The figure shows three views and two pictorial views of one solid part (mm, origin at its lowest corner). Answer the questions. A direction names the side the tool comes from. Give positions to 0.01 mm unless a question says otherwise; leave off trailing zeros. Loops run counter-clockwise (first coordinate to the right, second up) from the corner with the lowest first, then second, coordinate; pieces in that order, holes last. Notation, with made-up numbers: (35, 31.5) - (50, 31.5) arc R13 ccw to (50, 41.5) - close; hole circle Ø7 at (-28, -17). An arc over 180 degrees is marked (long way). Use a Markdown table: item, result. Add a question column.
Item 1: Which of the six approach directions +Z, -Z, +X, -X, +Y, -Y give full straight-line access (tool end or side, diameter ignored) to the marked faces 1, 2, 3, 4 and 5?
Item 2: Each of these flat-tipped pins is pushed along its axis until it touches: P1, Ø7.5, axis at x = 29, y = 15.5, coming from the +Z side; P2, Ø3, axis at y = 23, z = 4.5, coming from the +X side; P3, Ø8, axis at y = 25.5, z = 8, coming from the -X side (1 decimal); P4, Ø6.5, axis at x = 42.04, z = 10.16, coming from the -Y side. Where does it stop, or does it pass through?
Item 3: Consider probe 1 along X at (y, z) = (3.5, 10.16); probe 2 along X at (y, z) = (14.75, 16.75) (1 decimal); probe 3 along Y at (x, z) = (39, 16.5). Determine where each line is inside the solid, lowest interval first. Write a range as [from, to].
Item 4: A cutting plane is placed at B-B (x = 44.5). Determine the outline of the cut face in (y, z) (1 decimal), plus the area to 3 significant figures.
Item 5: For a pull along X with two mould halves and no side action, classify the marked faces 6, 7 and 8 as +X half, -X half, draft (parallel to the pull), parting line (faces both ways), or undercut.
Item 6: A cutting plane is placed at C-C (y = 14.25). Determine the outline of the cut face in (x, z) (1 decimal).
Item 7: A cutting plane is placed at D-D (z = 17). Determine the outline of the cut face in (x, y) (1 decimal).
Item 8: A cutting plane is placed at A-A (z = 9). Determine the outline of the cut face in (x, y) (1 decimal).
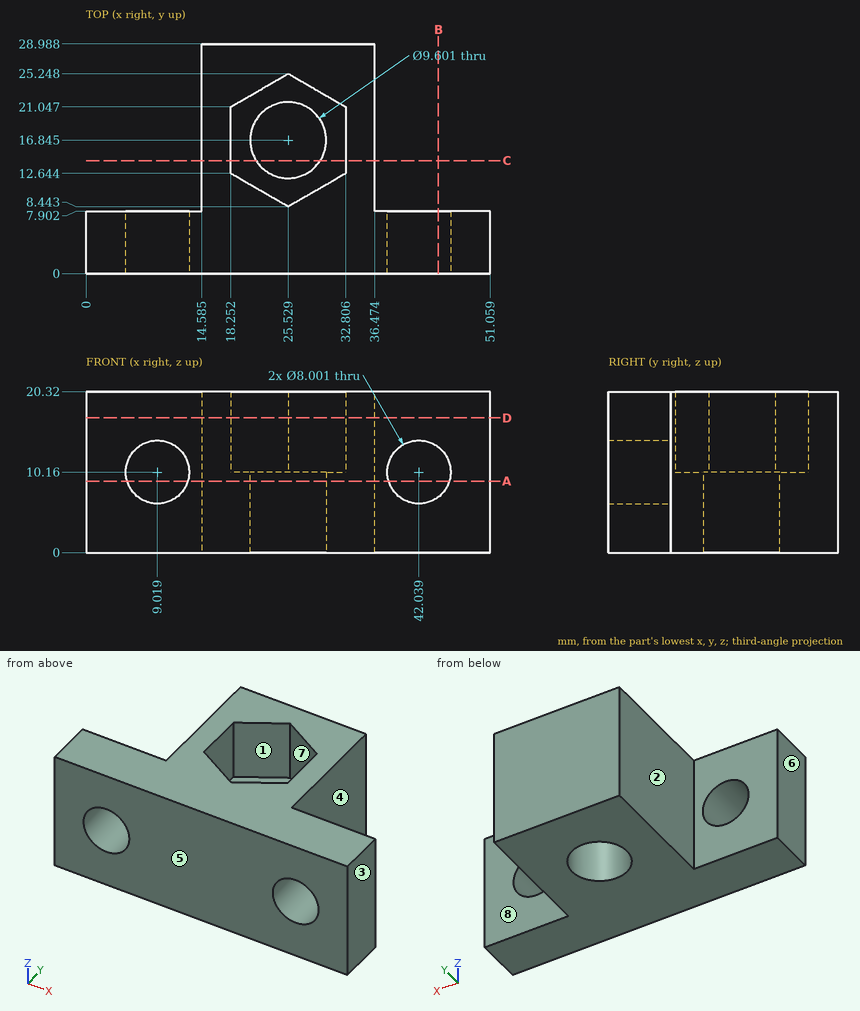
Geometry says:
| question | item | result |
|---|---|---|
| 1 | face 1 | +Z |
| 1 | face 2 | +Z, -Z, -X, +Y |
| 1 | face 3 | +Z, -Z, +X, +Y, -Y |
| 1 | face 4 | +Z, -Z, +X, +Y |
| 1 | face 5 | +Z, -Z, +X, -X, -Y |
| 2 | P1 | z = 10.16 |
| 2 | P2 | x = 36.47 |
| 2 | P3 | x = 14.6 |
| 2 | P4 | through |
| 3 | probe 1 | [0, 5.02], [13.02, 38.04], [46.04, 51.06] |
| 3 | probe 2 | [14.6, 18.3], [32.8, 36.5] |
| 3 | probe 3 | [0, 7.9] |
| 4 | outline | (0, 0) - (7.9, 0) - (7.9, 7) - (0, 7) - close; (0, 13.3) - (7.9, 13.3) - (7.9, 20.3) - (0, 20.3) - close |
| 4 | area | 111 mm² |
| 5 | face 6 | -X half |
| 5 | face 7 | undercut |
| 5 | face 8 | draft |
| 6 | outline | (14.6, 0) - (21.5, 0) - (21.5, 10.2) - (18.3, 10.2) - (18.3, 20.3) - (14.6, 20.3) - close; (29.6, 0) - (36.5, 0) - (36.5, 20.3) - (32.8, 20.3) - (32.8, 10.2) - (29.6, 10.2) - close |
| 7 | outline | (0, 0) - (51.1, 0) - (51.1, 7.9) - (36.5, 7.9) - (36.5, 29) - (14.6, 29) - (14.6, 7.9) - (0, 7.9) - close; hole (18.3, 12.6) - (25.5, 8.4) - (32.8, 12.6) - (32.8, 21) - (25.5, 25.2) - (18.3, 21) - close |
| 8 | outline | (0, 0) - (5.2, 0) - (5.2, 7.9) - (0, 7.9) - close; (12.8, 0) - (38.2, 0) - (38.2, 7.9) - (36.5, 7.9) - (36.5, 29) - (14.6, 29) - (14.6, 7.9) - (12.8, 7.9) - close; (45.9, 0) - (51.1, 0) - (51.1, 7.9) - (45.9, 7.9) - close; hole circle Ø9.6 at (25.5, 16.8) |
